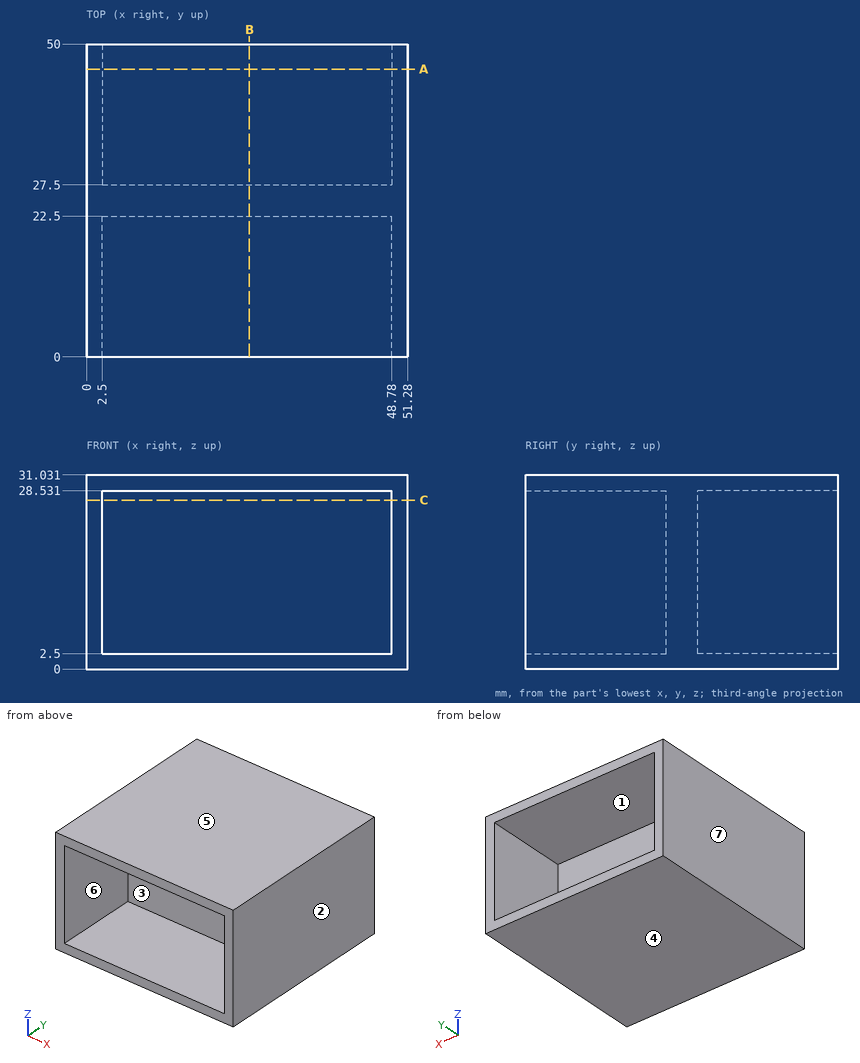
For this review, use the dimensioned drawing (mm, ordinates from the lowest corner) and the shaded views. A direction names the side the tool comes from. Coordinates: 2 decimals unless noted, no trailing zeros. Write each loop counter-clockwise with the first axis right and the second up, starting at its lowest first coordinate (ties: lowest second). Pieces come first, ordered by that corner, then holes. Notation, with made-up numbers: (-28, 19) - (-13, 19) arc R4 ccw to (-13, 25) - close; hole circle Ø4 at (-30.75, -37). An arc over 180 degrees is marked (long way). Answer in a Markdown table with one row per item. Add a question column.
Q1. For the marked faces 1, 2 and 3, list the 3-axis set-ups (+Z, -Z, +X, -X, +Y, -Y) from which the entire face can be reached by the end or side of a thin tool; tool diameter is ignored.
Q2. Clearance check with flat-ended pins moving along their axes: pin 1 (3 mm diameter, centred on x = 15, z = 22.5, fed in from +Y); pin 2 (8 mm diameter, centred on x = 18, z = 19.5, fed in from -Y). State where each tip first meets the part, or that it passes through.
Q3. Consider section B-B on x = 26. Give the boundary of the cut face in (y, z).
Q4. Draft analysis for pull direction Z (two halves, no side actions). For the marked faces 4, 5, 6 and 7, state which applies: +Z half, -Z half, draft (parallel to the pull), parting line (faces both ways), or undercut.
Q5. Consider section A-A on y = 46. Give the boundary of the cut face in (x, z).
Q6. Consider section C-C on z = 27. Give the boundary of the cut face in (x, y).
Q7. To check wall thickness, follow line 1 along X through (y, z) = (19, 18.5); line 2 along Z through (x, y) = (46, 31); line 3 along Y through (x, z) = (38.5, 8). State the ranges of each line that lie inside material, in increasing order. Write a range as from..to.
Answers below:
| question | item | result |
|---|---|---|
| 1 | face 1 | +Y |
| 1 | face 2 | +Z, -Z, +X, +Y, -Y |
| 1 | face 3 | -Y |
| 2 | pin 1 | y = 27.5 |
| 2 | pin 2 | y = 22.5 |
| 3 | outline | (0, 0) - (50, 0) - (50, 2.5) - (27.5, 2.5) - (27.5, 28.53) - (50, 28.53) - (50, 31.03) - (0, 31.03) - (0, 28.53) - (22.5, 28.53) - (22.5, 2.5) - (0, 2.5) - close |
| 4 | face 4 | -Z half |
| 4 | face 5 | +Z half |
| 4 | face 6 | undercut |
| 4 | face 7 | draft |
| 5 | outline | (0, 0) - (51.28, 0) - (51.28, 31.03) - (0, 31.03) - close; hole (2.5, 2.5) - (48.78, 2.5) - (48.78, 28.53) - (2.5, 28.53) - close |
| 6 | outline | (0, 0) - (2.5, 0) - (2.5, 22.5) - (48.78, 22.5) - (48.78, 0) - (51.28, 0) - (51.28, 50) - (48.78, 50) - (48.78, 27.5) - (2.5, 27.5) - (2.5, 50) - (0, 50) - close |
| 7 | line 1 | 0..2.5, 48.78..51.28 |
| 7 | line 2 | 0..2.5, 28.53..31.03 |
| 7 | line 3 | 22.5..27.5 |
